from build123d import *

# Parameters (mm, degrees)
SKETCH2_W           = 33
SKETCH2_H           = 27
BOSS_EXTRUDE1_DEPTH = 20
CUT_EXTRUDE1_DEPTH  = 18
BOSS_EXTRUDE3_DEPTH = 25
CUT_EXTRUDE4_DEPTH  = 2
SKETCH10_W          = 2
SKETCH10_H          = 5
BOSS_EXTRUDE4_DEPTH = 5
SKETCH11_W          = 2
SKETCH11_H          = 5
BOSS_EXTRUDE5_DEPTH = 5
SKETCH12_R          = 1.25
CUT_EXTRUDE5_DEPTH  = 2


with BuildPart() as part:
    # Sketch2 → Boss-Extrude1 (new body)
    with BuildSketch(Plane.XY):
        Rectangle(SKETCH2_W, SKETCH2_H)
    extrude(amount=-BOSS_EXTRUDE1_DEPTH)

    # Sketch3 → Cut-Extrude1 (cut)
    with BuildSketch(Plane(origin=(0, 0, -20), x_dir=(-1, 0, 0), z_dir=(0, 0, -1))):
        with BuildLine():
            Line((-14.5, 11), (-14.5, -11))
            Line((-14.5, -11), (14.5, -11))
            Line((14.5, -11), (14.5, 11))
            add(Edge.make_bspline(
                [(-14.5, 11), (0, 13), (14.5, 11)],
                knots=[0, 0, 0, 1, 1, 1], degree=2))
        make_face()
    extrude(amount=-CUT_EXTRUDE1_DEPTH, mode=Mode.SUBTRACT)

    # Sketch4 → Boss-Extrude3 (add)
    with BuildSketch(Plane(origin=(0, 13.5, 0), x_dir=(1, 0, 0), z_dir=(0, 1, 0))):
        with BuildLine():
            Line((14.504051414, 5), (14.504051414, 2))
            Line((14.504051414, 2), (14.504051414, 1))
            Line((14.504051414, 1), (10.553086369, 1))
            add(Edge.make_bspline(
                [(14.504051414, 5), (13.626897644, 2.036892848), (10.553086369, 1)],
                knots=[0, 0, 0, 1, 1, 1], degree=2))
        make_face()
        with BuildLine():
            add(Edge.make_bspline(
                [(-14.504051414, 5), (-13.626897644, 2.036892848), (-10.553086369, 1)],
                knots=[0, 0, 0, 1, 1, 1], degree=2))
            Line((-10.553086369, 1), (-14.504051414, 1))
            Line((-14.504051414, 1), (-14.504051414, 2))
            Line((-14.504051414, 2), (-14.504051414, 5))
        make_face()
    extrude(amount=-BOSS_EXTRUDE3_DEPTH)

    # Sketch9 → Cut-Extrude4 (cut)
    with BuildSketch(Plane(origin=(0, 0, -2), x_dir=(-1, 0, 0), z_dir=(0, 0, -1))):
        with BuildLine():
            Line((-12.486551431, 11.258435355), (-12.486551431, -11))
            Line((-12.486551431, -11), (12.486551431, -11))
            Line((12.486551431, -11), (12.486551431, 11.258435355))
            add(Edge.make_bspline(
                [(-12.486551431, 11.258435355), (0, 12.741564645), (12.486551431, 11.258435355)],
                knots=[0, 0, 0, 1, 1, 1], degree=2))
        make_face()
    extrude(amount=-CUT_EXTRUDE4_DEPTH, mode=Mode.SUBTRACT)

    # Sketch10 → Boss-Extrude4 (add)
    with BuildSketch(Plane.ZY.offset(16.5)):
        with Locations((-4, 7)):
            Rectangle(SKETCH10_W, SKETCH10_H)
        with Locations((-4, -7)):
            Rectangle(SKETCH10_W, SKETCH10_H)
    extrude(amount=BOSS_EXTRUDE4_DEPTH)

    # Sketch11 → Boss-Extrude5 (add)
    with BuildSketch(Plane(origin=(16.5, 0, 0), x_dir=(0, 0, -1), z_dir=(1, 0, 0))):
        with Locations((4, 7)):
            Rectangle(SKETCH11_W, SKETCH11_H)
        with Locations((4, -7)):
            Rectangle(SKETCH11_W, SKETCH11_H)
    extrude(amount=BOSS_EXTRUDE5_DEPTH)

    # Sketch12 → Cut-Extrude5 (cut)
    with BuildSketch(Plane.XY.offset(-3)):
        with Locations((19, -7)):
            Circle(SKETCH12_R)
        with Locations((19, 7)):
            Circle(SKETCH12_R)
        with Locations((-19, 7)):
            Circle(SKETCH12_R)
        with Locations((-19, -7)):
            Circle(SKETCH12_R)
    extrude(amount=-CUT_EXTRUDE5_DEPTH, mode=Mode.SUBTRACT)


solid = part.part
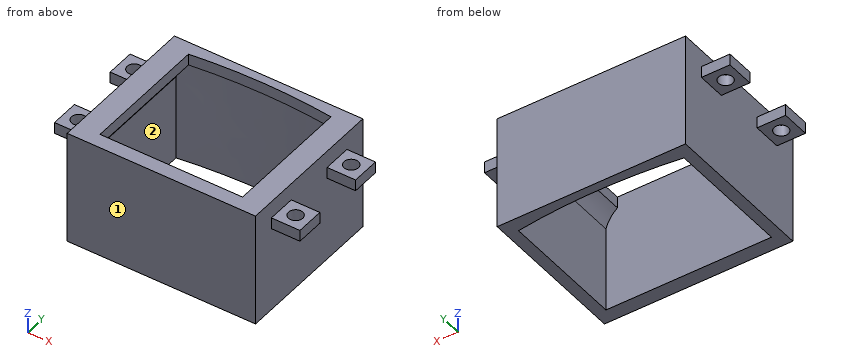
Read the model definition and answer for the solid it produces. Units are mm, in the model's axes. Face numbers are marked on the shaded views. A direction names the side the tool comes from. Give positions to 0.01 mm unless a question says otherwise; leave off trailing zeros. Write each loop counter-clockwise with the first axis right and the second up, starting at its lowest first coordinate (ties: lowest second). Pieces come first, ordered by that corner, then holes. Notation, with made-up numbers: M -27.5,57 L 14.5,57 A29 cw 14.5,94 Z; hole C -25,-3 d5. An arc over 180 degrees is marked long. One line per item, written item: value. Start each with the question number.
(1) Find section B-B (y = -7). Give the number of separate pieces and of enclosed holes in the cut face, plus the area to 3 significant figures.
(2) A tool of negligible diameter and unlimited length cuts with its end or side. For the marked faces 1 and 2, from which of +Z, -Z, +X, -X, +Y, -Y can it reach the whole face along a straight path? Write none if from no direction.
(3) Find section A-A (x = 19). Determine the outline of the cut face in (y, z), plus the area to 3 significant figures.
(4) Flat-ended cylindrical pins translate along their axes: pin 1 Ø3 at (x, y) = (19, -7) entering from +Z; pin 2 Ø0.6 at (x, z) = (19, -4) entering from +Y; pin 3 Ø2 at (x, z) = (18.5, -4) entering from -Y. Find the tip coordinate at first contact, or state that the pin passes through.
(5) Find the intervals of material crossed by line 1 (Y direction, x = 19, z = -4.5); line 2 (X direction, y = 7.75, z = -18.75); line 3 (Y direction, x = 12.5, z = -15), in increasing order.
Results below:
1. separate pieces: 4
1. enclosed holes: 0
1. area: 103 mm^2
2. face 1: +Z, -Z, +X, -X, -Y
2. face 2: -Z
3. outline: M -9.5,-5 L -8.25,-5 L -8.25,-3 L -9.5,-3 Z; M -5.75,-5 L -4.5,-5 L -4.5,-3 L -5.75,-3 Z; M 4.5,-5 L 5.75,-5 L 5.75,-3 L 4.5,-3 Z; M 8.25,-5 L 9.5,-5 L 9.5,-3 L 8.25,-3 Z
3. area: 10.0 mm^2
4. pin 1: stops at z = -3
4. pin 2: stops at y = 9.5
4. pin 3: stops at y = -9.5
5. line 1: y = -9.5 to -8.25, -5.75 to -4.5, 4.5 to 5.75, 8.25 to 9.5
5. line 2: x = -16.5 to -14.5, 14.5 to 16.5
5. line 3: y = -13.5 to -11, 11.26 to 13.5
